Input: part model. Units: mm. Frame: model coordinates. A direction names the side the tool comes from. Give positions to 0.01 mm unless a question says otherwise; leave off trailing zeros. Order: outer loops, then holes, each group sorted by start corner. A loop starts at its lowest first (then second) coordinate and runs counter-clockwise, first axis right, second up. Notation, with made-up numbers: (25.25, 89) - (63.25, 89) arc R23 ccw to (63.25, 111) - close; hole circle Ø4 at (6.5, 23.25). An arc over 180 degrees is marked (long way). Use a Markdown table: item, result.
from build123d import *

# Parameters (mm, degrees)
BOSS_EXTRUDE1_DEPTH = 37
SKETCH3_R           = 10.25
SKETCH3_R_2         = 1.05
SKETCH3_R_3         = 3.79119947
CUT_EXTRUDE1_DEPTH  = 38
CUT_EXTRUDE5_DEPTH  = 35
SKETCH10_R          = 1.05
CUT_EXTRUDE6_DEPTH  = 35
SKETCH15_W          = 15.770937014
SKETCH15_H          = 5.000421699
CUT_EXTRUDE8_DEPTH  = 35
SKETCH17_W          = 10.43544962
SKETCH17_H          = 35
CUT_EXTRUDE10_DEPTH = 38


with BuildPart() as part:
    # Sketch1 → Boss-Extrude1 (new body)
    with BuildSketch(Plane(origin=(0, 0, 0), x_dir=(1, 0, 0), z_dir=(0, 1, 0))):
        with BuildLine():
            Line((30.91362152, -11.506988518), (61.410209359, 36.471719739))
            ThreePointArc((61.410209359, 36.471719739), (65.035248289, 39.872184028), (69.84963689, 41.10738726))
            Line((69.84963689, 41.10738726), (230.684249594, 41.10738726))
            ThreePointArc((230.684249594, 41.10738726), (235.498638195, 39.872184028), (239.123677125, 36.471719739))
            Line((239.123677125, 36.471719739), (269.620264964, -11.506988518))
            ThreePointArc((269.620264964, -11.506988518), (270.941569742, -19.045741561), (266.545169913, -25.310748528))
            Line((266.545169913, -25.310748528), (256.707586966, -31.563787081))
            ThreePointArc((256.707586966, -31.563787081), (249.168833923, -32.885091859), (242.903826956, -28.488692029))
            Line((242.903826956, -28.488692029), (219.802518103, 7.855405338))
            ThreePointArc((219.802518103, 7.855405338), (216.177479173, 11.255869627), (211.363090572, 12.491072858))
            Line((211.363090572, 12.491072858), (89.170795912, 12.491072858))
            ThreePointArc((89.170795912, 12.491072858), (84.356407311, 11.255869627), (80.731368381, 7.855405338))
            Line((80.731368381, 7.855405338), (57.630059528, -28.488692029))
            ThreePointArc((57.630059528, -28.488692029), (51.365052561, -32.885091859), (43.826299518, -31.563787081))
            Line((43.826299518, -31.563787081), (33.988716571, -25.310748528))
            ThreePointArc((33.988716571, -25.310748528), (29.592316741, -19.045741561), (30.91362152, -11.506988518))
        make_face()
    extrude(amount=BOSS_EXTRUDE1_DEPTH)

    # Sketch3 → Cut-Extrude1 (cut, through all)
    with BuildSketch(Plane(origin=(0, 37, 0), x_dir=(1, 0, 0), z_dir=(0, 1, 0))):
        with Locations((255.189179464, -18.309954767)):
            Circle(SKETCH3_R)
        with Locations((259.912867141, -5.235675639)):
            Circle(SKETCH3_R_2)
        with Locations((241.346126573, -17.037207093)):
            Circle(SKETCH3_R_2)
        with Locations((45.34470702, -18.309954767)):
            Circle(SKETCH3_R_3)
    extrude(amount=-CUT_EXTRUDE1_DEPTH, mode=Mode.SUBTRACT)

    # Sketch9 → Cut-Extrude5 (cut)
    with BuildSketch(Plane.XZ):
        Polygon((220.770453038, -9.128850504), (250.101424494, 37.016053635), (274.286034243, 21.643649867), (245.369620358, -23.849052233), align=None)
    extrude(amount=-CUT_EXTRUDE5_DEPTH, mode=Mode.SUBTRACT)

    # Sketch10 → Cut-Extrude6 (cut)
    with BuildSketch(Plane(origin=(186.824736014, 0, -118.750945563), x_dir=(-0.536433248, 0, -0.843942753), z_dir=(0.843942753, 0, -0.536433248))):
        with Locations((-148.344514011, 24)):
            Circle(SKETCH10_R)
        with Locations((-148.344514011, 12)):
            Circle(SKETCH10_R)
        with Locations((-124.344514011, 12)):
            Circle(SKETCH10_R)
        with Locations((-124.344514011, 24)):
            Circle(SKETCH10_R)
    extrude(amount=-CUT_EXTRUDE6_DEPTH, mode=Mode.SUBTRACT)

    # Sketch15 → Cut-Extrude8 (cut)
    with BuildSketch(Plane(origin=(160.108298005, 0, -101.769242052), x_dir=(0.536433248, 0, 0.843942753), z_dir=(-0.843942753, 0, 0.536433248))):
        with Locations((134.025974507, 2.50021085)):
            Rectangle(SKETCH15_W, SKETCH15_H)
    extrude(amount=-CUT_EXTRUDE8_DEPTH, mode=Mode.SUBTRACT)

    # Sketch17 → Cut-Extrude10 (cut)
    with BuildSketch(Plane(origin=(160.108298005, 0, -101.769242052), x_dir=(0.536433248, 0, 0.843942753), z_dir=(-0.843942753, 0, 0.536433248))):
        with Locations((159.562238821, 17.5)):
            Rectangle(SKETCH17_W, SKETCH17_H)
    extrude(amount=-CUT_EXTRUDE10_DEPTH, mode=Mode.SUBTRACT)


solid = part.part
1. Section query C-C (x = 223). Return loops of the section in (y, z), then the cut area to 3 significant figures.
Response:
| item | result |
|---|---|
| outline | (0, -41.11) - (37, -41.11) - (37, -2.82) - (0, -2.82) - (0, -5.62) - (35, -5.62) - (35, -10.46) - (0, -10.46) - close |
| area | 1,250 mm^2 |
2. Pin query (flat end, axial travel): pin 1 (5 mm diameter, centred on x = 231.5, z = 8, fed in from -Y); pin 2 (2 mm diameter, centred on x = 246.5, y = 26, fed in from +Z); pin 3 (8 mm diameter, centred on y = 31, z = -30.5, fed in from -X). Return the tip coordinate at first contact, or that it passes through.
Response:
| item | result |
|---|---|
| pin 1 | stops at y = 5 |
| pin 2 | stops at z = -20.5 |
| pin 3 | stops at x = 55.07 |
3. Section query A-A (z = -2). Return loops of the section in (x, y).
Response:
| item | result |
|---|---|
| outline | (39.5, 0) - (77.01, 0) - (77.01, 37) - (39.5, 37) - close; (223.52, 0) - (225.3, 0) - (225.3, 35) - (259.26, 35) - (259.26, 5) - (261.03, 5) - (261.03, 37) - (223.52, 37) - close |
4. Section query B-B (y = 19.5). Return loops of the section in (x, z), then the cut area to 3 significant figures.
Response:
| item | result |
|---|---|
| outline | (30.91, 11.51) - (61.41, -36.47) arc R10 ccw to (69.85, -41.11) - (230.68, -41.11) arc R10 ccw to (239.12, -36.47) - (269.62, 11.51) - (268.35, 12.31) - (245.37, -23.85) - (220.77, -9.13) - (244.17, 27.68) - (242.9, 28.49) - (219.8, -7.86) arc R10 cw to (211.36, -12.49) - (89.17, -12.49) arc R10 cw to (80.73, -7.86) - (57.63, 28.49) arc R10 ccw to (43.83, 31.56) - (33.99, 25.31) arc R10 ccw to start; hole circle Ø7.58 at (45.34, 18.31) |
| area | 6,860 mm^2 |
5. Section query D-D (z = -33.5). Return loops of the section in (x, y), then the cut area to 3 significant figures.
Response:
| item | result |
|---|---|
| outline | (59.52, 0) - (241.01, 0) - (241.01, 37) - (59.52, 37) - close |
| area | 6,720 mm^2 |
6. Set-up query: faces 1 (the face through (257.02, 17.26, -5.52)), 2 (the face through (38.976, 18.241, 28.481)), 3 (the face through (149, 18, -41.107)), 4 (the face through (216.24, 18.24, -11.22)), 5 (the face through (246, 35, -1)). Return all of +Z, -Z, +X, -X, +Y, -Y with unobstructed straight access to the full face (end or side cutting, diameter ignored); none if empty.
Response:
| item | result |
|---|---|
| face 1 | +Z, -Y |
| face 2 | +Z, -X, +Y, -Y |
| face 3 | -Z, +X, -X, +Y, -Y |
| face 4 | +Z, +Y, -Y |
| face 5 | -Y |
7. Material intervals for line 1 along X through (y, z) = (14.5, 3.5); line 2 along X through (y, z) = (17.5, -3); line 3 along X through (y, z) = (3, -15.5), sorted ascending.
Response:
| item | result |
|---|---|
| line 1 | x = 36 to 73.51, 227.02 to 228.8, 262.75 to 264.53 |
| line 2 | x = 40.13 to 77.65, 222.89 to 224.67, 258.62 to 260.4 |
| line 3 | x = 48.08 to 231.42, 250.68 to 252.45 |
8. Mould query, pull axis X, two halves, no side actions, for faces 6 (the face through (118, 0, -21)), 7 (the face through (48.847, 18.759, 19.762)), 8 (the face through (254.158, 18.241, -12.818)). Classes: pulls with the +X half, pulls with the -X half, needs draft (parallel to the pull), parting line crosses it, or undercut.
Response:
| item | result |
|---|---|
| face 6 | needs draft |
| face 7 | undercut |
| face 8 | pulls with the +X half |
